Work out the finished part from the listing and answer in its coordinate system (mm). Coordinates: 2 decimals unless noted, no trailing zeros. Loops run counter-clockwise (first coordinate to the right, second up) from the corner with the lowest first, then second, coordinate; pieces in that order, holes last. Notation, with made-up numbers: (63, 23.5) - (116, 23.5) arc R19 ccw to (116, 56.5) - close; hole circle Ø3 at (-36.5, 40). An arc over 180 degrees is marked (long way). Write each question's results on one line, items separated by ' | '. Start each with the question number.
1. Find the intervals of material crossed by line 1 along X through (y, z) = (0.2, -7) (3 decimals); line 2 along Y through (x, z) = (5, 0) (3 decimals); line 3 along Z through (x, y) = (7.25, 0.2), in increasing order. Write a range as [from, to].
2. A cutting plane is placed at A-A on x = -7. Determine the outline of the cut face in (y, z) (3 decimals), then the cut area to 3 significant figures.
3. Each of these flat-tipped pins is pushed along its axis until it touches: P1, Ø2.5, axis at x = -7.505, z = -7.315, coming from the +Y side; P2, Ø5, axis at x = -5, z = 4.5, coming from the -Y side (3 decimals); P3, Ø10, axis at x = -4.5, z = -3, coming from the -Y side (3 decimals). Where does it stop, or does it pass through?
4. A cutting plane is placed at B-B on z = -8. Determine the outline of the cut face in (x, y) (3 decimals).
5. A cutting plane is placed at C-C on z = 0.75. Determine the outline of the cut face in (x, y) (3 decimals), then the cut area to 3 significant figures.
6. A cutting plane is placed at D-D on y = -0.35. Determine the outline of the cut face in (x, z) (3 decimals).
from build123d import *

# Parameters (mm, degrees)
SKETCH1_W               = 20.38
SKETCH1_H               = 20
BOSS_EXTRUDE1_DEPTH     = 0.775
CUT_EXTRUDE1_DEPTH      = 15.361009714
CUT_EXTRUDE1_DEPTH_BACK = 15.361009714
SKETCH2_R               = 1.435
FILLET1_R               = 1
SKETCH3_W               = 2
SKETCH3_H               = 2.56
BOSS_EXTRUDE2_DEPTH     = 0.5


with BuildPart() as part:
    # Sketch1 → Boss-Extrude1 (new, symmetric)
    with BuildSketch(Plane(origin=(0, 0, 0), x_dir=(1, 0, 0), z_dir=(0, 1, 0))):
        Rectangle(SKETCH1_W, SKETCH1_H)
    extrude(amount=BOSS_EXTRUDE1_DEPTH, both=True)

    # Sketch2 → Cut-Extrude1 (cut, two sides: drawn at the far end of the back side and taken through both)
    with BuildSketch(Plane(origin=(0, 0.775, 0), x_dir=(1, 0, 0), z_dir=(0, 1, 0)).offset(-CUT_EXTRUDE1_DEPTH_BACK)):
        with Locations(Location((-7.505, 7.315, 0), (0, 0, 270))):
            Circle(SKETCH2_R)
        with Locations(Location((7.505, 7.315, 0), (0, 0, 270))):
            Circle(SKETCH2_R)
    extrude(amount=CUT_EXTRUDE1_DEPTH + CUT_EXTRUDE1_DEPTH_BACK, mode=Mode.SUBTRACT)

    # Fillet1
    fillet1_edges = [part.edges().sort_by_distance(p)[0] for p in [
        (10.19, 0, 10),
        (-10.19, 0, 10),
        (-10.19, 0, -10),
        (10.19, 0, -10),
    ]]
    fillet(fillet1_edges, radius=FILLET1_R)

    # Sketch3 → Boss-Extrude2 (add)
    with BuildSketch(Plane(origin=(0, -0.775, 0), x_dir=(-1, 0, 0), z_dir=(0, -1, 0))):
        Rectangle(SKETCH3_W, SKETCH3_H)
    extrude(amount=BOSS_EXTRUDE2_DEPTH)


solid = part.part
Values:
1) line 1: [-10.19, -8.905], [-6.105, 6.105], [8.905, 10.19] | line 2: [-0.775, 0.775] | line 3: [-10, -8.73], [-5.9, 10]
2) outline: (-0.775, -10) - (0.775, -10) - (0.775, -8.658) - (-0.775, -8.658) - close; (-0.775, -5.972) - (0.775, -5.972) - (0.775, 10) - (-0.775, 10) - close | area: 26.8 mm^2
3) P1: through | P2: y = -0.775 | P3: y = -1.275
4) outline: (-10.19, -0.775) - (-8.766, -0.775) - (-8.766, 0.775) - (-10.19, 0.775) - close; (-6.244, -0.775) - (6.244, -0.775) - (6.244, 0.775) - (-6.244, 0.775) - close; (8.766, -0.775) - (10.19, -0.775) - (10.19, 0.775) - (8.766, 0.775) - close
5) outline: (-10.19, -0.775) - (-1, -0.775) - (-1, -1.275) - (1, -1.275) - (1, -0.775) - (10.19, -0.775) - (10.19, 0.775) - (-10.19, 0.775) - close | area: 32.6 mm^2
6) outline: (-10.19, -9) arc R1 ccw to (-9.19, -10) - (9.19, -10) arc R1 ccw to (10.19, -9) - (10.19, 9) arc R1 ccw to (9.19, 10) - (-9.19, 10) arc R1 ccw to (-10.19, 9) - close; hole circle Ø2.87 at (-7.505, -7.315); hole circle Ø2.87 at (7.505, -7.315)
